Autodesk Inventor part; units mm, degrees
ref_plane "Work Plane1" through (29, 4.15, 0) normal (1, 0, 0) x (0, 0, -1)
ref_plane "YZ Plane" through (0, 0, 0) normal (1, 0, 0) x (0, 1, 0)
ref_plane "XZ Plane" through (0, 0, 0) normal (0, 1, 0) x (-1, 0, 0)
sketch "Sketch5" plane through (0, 0, 0) normal (0, 0, 1) x (1, 0, 0)
  line L0 (0, 0) -> (20, 0)
  line L1 (20, 0) -> (20, 10)
  line L2 (20, 10) -> (0, 10)
  line L3 (0, 10) -> (0, 0)
  line L4 (20, 4.15) -> (30, 4.15)
  line L5 (30, 4.15) -> (30, 5.85)
  line L6 (30, 5.85) -> (20, 5.85)
  line L7 (20, 5.85) -> (20, 4.15)
  point P0 (20, 5)
  point P1 (20, 5)
  dimension "d11" = 10
  dimension "d12" = 1.7
  dimension "d13" = 20
  dimension "d14" = 10
extrude "Extrusion3" add sketch "Sketch5" along normal blind 0.5
chamfer "Chamfer1" distance 3 angle 45 2 edges at (20, 10, 0.25) (20, 0, 0.25)
ref_plane "Work Plane1" through (29, 4.15, 0) normal (1, 0, 0) x (0, 0, -1)
sketch "Sketch6" plane through (29, 4.15, 0) normal (1, 0, 0) x (0, 0, -1)
  line L0 (0, 1.7) -> (0, 0)
  line L1 (0, 0) -> (-0.5, 0)
  line L2 (-0.5, 0) -> (-0.5, 1.7)
  line L3 (-0.5, 1.7) -> (0, 1.7)
  arc A0 (-0.5, 1.7) -> (-0.5, 0) centre (-0.5, 0.85) ccw
  point P0 (0, -4.15)
extrude "Extrusion4" add sketch "Sketch6" against normal up to surface (29 mm away) contours L2 A0
properties part number "current-adjusting-screwdriver"
CAD build for the part. Positions are in the model's coordinates, mm. A direction names the side the tool comes from. Round coordinates to 2 decimals unless told otherwise and drop trailing zeros. Write each loop counter-clockwise with the first axis right and the second up, starting at its lowest first coordinate (ties: lowest second). Pieces come first, ordered by that corner, then holes. Notation, with made-up numbers: (81.25, 88) -> (140.25, 88) arc R28 ccw to (140.25, 110) -> close; hole circle Ø11 at (36.25, 83). An arc over 180 degrees is marked (long way). Answer in a Markdown table with one row per item. Add a question column.
Item 1: Saw through at C-C, the plane x = 8.25. Write the cut outline in (y, z).
Item 2: Drill centre lines: line 1 (Z direction, x = 15, y = 8.75); line 2 (Y direction, x = 28, z = 0.55); line 3 (X direction, y = 6.75, z = 0.1). Where is each one in solid material? Low to high. Write a range as from..to.
Item 3: Saw through at B-B, the plane y = 1. Write the cut outline in (x, z), then the cut area to 3 significant figures.
Item 4: Saw through at A-A, the plane z = 0.25. Write the cut outline in (x, y), then the cut area to 3 significant figures.
Item 5: Saw through at D-D, the plane y = 5.5. Write the cut outline in (x, z), then the cut area to 3 significant figures.
Item 6: Drop flat-ended pins along their axis: pin 1 Ø0.6 at (x, z) = (22.5, 0.5) entering from -Y; pin 2 Ø1.2 at (x, y) = (9.5, 1) entering from +Z. Give the stop position or say it passes through.
Item 7: Which spindle directions (+Z, -Z, +X, -X, +Y, -Y) get a long thin tool onto all of the face, cutting with end or side? Do faces 1 (the face through (10, 2, 0.5)), 2 (the face through (10, 8, 0.5)), 3 (the face through (29, 5, 1)). Say none if no direction does.
Findings below:
| question | item | result |
|---|---|---|
| 1 | outline | (0, 0) -> (10, 0) -> (10, 0.5) -> (5.85, 0.5) arc R0.85 ccw to (4.15, 0.5) -> (0, 0.5) -> close |
| 2 | line 1 | z = 0..0.5 |
| 2 | line 2 | y = 4.15..5.85 |
| 2 | line 3 | x = 0..20 |
| 3 | outline | (0, 0) -> (18, 0) -> (18, 0.5) -> (0, 0.5) -> close |
| 3 | area | 9.00 mm^2 |
| 4 | outline | (0, 0) -> (17, 0) -> (20, 3) -> (20, 4.15) -> (30, 4.15) -> (30, 5.85) -> (20, 5.85) -> (20, 7) -> (17, 10) -> (0, 10) -> close |
| 4 | area | 208 mm^2 |
| 5 | outline | (0, 0) -> (30, 0) -> (30, 0.5) -> (29, 0.5) -> (29, 1.19) -> (0, 1.19) -> close |
| 5 | area | 34.9 mm^2 |
| 6 | pin 1 | stops at y = 4.15 |
| 6 | pin 2 | stops at z = 0.5 |
| 7 | face 1 | +Z, +X, -X, -Y |
| 7 | face 2 | +Z, +X, -X, +Y |
| 7 | face 3 | +Z, +X, +Y, -Y |
